```python
from build123d import *

# Parameters (mm, degrees)
F1_DEPTH = 25
F2_W     = 15
F2_H     = 7.5
F3_DEPTH = 25


with BuildPart() as f1:
    # F0 (on Front) → F1 (new body)
    with BuildSketch(Plane.XZ):
        Polygon((0, 400), (0, 385), (200, 385), (267.885888, 0), (282.885888, 0), (207.065286, 430), (192.065286, 430), (197.355095, 400), align=None)
        Polygon((-207.065286, 430), (-282.885888, 0), (-267.885888, 0), (-200, 385), (0, 385), (0, 400), (-197.355095, 400), (-192.065286, 430), align=None)
    extrude(amount=F1_DEPTH)

    # F2 (on face) → F3 (cut, through all)
    with BuildSketch(Plane.XZ.offset(25)):
        with Locations((0, 388.75)):
            Rectangle(F2_W, F2_H)
    extrude(amount=-F3_DEPTH, mode=Mode.SUBTRACT)


solid = f1.part
```
Design review of the part built by this model. Coordinates are the model's own, in mm. A direction names the side the tool comes from. Round coordinates to 2 decimals unless told otherwise and drop trailing zeros. Write each loop counter-clockwise with the first axis right and the second up, starting at its lowest first coordinate (ties: lowest second). Pieces come first, ordered by that corner, then holes.
Item 1: We need section D-D on x = -234. Write out the cut boundary in (y, z), and give its area (3 significant figures).
Item 2: We need section A-A on z = 217.5. Write out the cut boundary in (x, y), and give its area (3 significant figures).
Item 3: The part is to be moulded in two halves that separate along Z. For faces 4 (the flat face through (-244.445, -12.325, 218.01)), 5 (the flat face through (20, -25, 391)), 6 (the flat face through (-194.747, -12.325, 414.79)), say which applies: +Z half, -Z half, draft (parallel to the pull), parting line (faces both ways), or undercut.
Item 4: For probe 1 along Z at (x, y) = (-20.5, -4.25); probe 2 along X at (y, z) = (-20.5, 368); probe 3 along X at (y, z) = (-8.5, 248), list the stretches that pass through material, from the lowest coordinate up.
Item 5: We need section C-C on x = 128.5. Write out the cut boundary in (y, z), and give its area (3 significant figures).
Item 6: For faces 1 (the flat face through (0, -13, 392.5)), 2 (the flat face through (194.673, -12.325, 415.21)), 3 (the flat face through (245.506, -12.325, 211.99)), list the 3-axis set-ups (+Z, -Z, +X, -X, +Y, -Y) from which the entire face can be reached by the end or side of a thin tool; tool diameter is ignored.
Item 7: We need section B-B on y = -16.75. Write out the cut boundary in (x, z).
Item 8: Clearance check with flat-ended pins moving along their axes: pin 1 Ø12 at (y, z) = (-6, 204.5) entering from -X (3 decimals); pin 2 Ø8 at (y, z) = (-14.5, 390) entering from -X; pin 3 Ø10 at (y, z) = (-21, 260.5) entering from -X. State where each tip first meets the part, or that it passes through.
Returned:
1. outline: (-25, 192.18) - (0, 192.18) - (0, 277.25) - (-25, 277.25) - close
1. area: 2,130 mm2
2. outline: (-244.53, -25) - (-229.53, -25) - (-229.53, 0) - (-244.53, 0) - close; (229.53, -25) - (244.53, -25) - (244.53, 0) - (229.53, 0) - close
2. area: 750 mm2
3. face 4: +Z half
3. face 5: draft
3. face 6: undercut
4. probe 1: z = 385 to 400
4. probe 2: x = -218 to -203, 203 to 218
4. probe 3: x = -239.16 to -224.16, 224.16 to 239.16
5. outline: (-25, 385) - (0, 385) - (0, 400) - (-25, 400) - close
5. area: 375 mm2
6. face 1: -Z, +Y, -Y
6. face 2: +Y, -Y
6. face 3: +Z, +X, +Y, -Y
7. outline: (-282.89, 0) - (-267.89, 0) - (-200, 385) - (-7.5, 385) - (-7.5, 392.5) - (7.5, 392.5) - (7.5, 385) - (200, 385) - (267.89, 0) - (282.89, 0) - (207.07, 430) - (192.07, 430) - (197.36, 400) - (-197.36, 400) - (-192.07, 430) - (-207.07, 430) - close
8. pin 1: stops at x = -247.885
8. pin 2: stops at x = -214.82
8. pin 3: stops at x = -237.83
